```python
from build123d import *

# Parameters (mm, degrees)
SKETCH1_R           = 5
SKETCH1_R_2         = 3
SKETCH1_W           = 45.892135624
SKETCH1_H           = 6.35
BOSS_EXTRUDE1_DEPTH = 6.35
SKETCH2_R           = 1.5
CUT_EXTRUDE1_DEPTH  = 28.889427262


with BuildPart() as part:
    # Sketch1 → Boss-Extrude1 (new body)
    # profile 1 of 5: a face of its own
    with BuildSketch(Plane.XY):
        Circle(SKETCH1_R)
        Circle(SKETCH1_R_2, mode=Mode.SUBTRACT)
    # profile 2 of 5: a face of its own
    with BuildSketch(Plane.XY):
        with BuildLine():
            ThreePointArc((-4.582078525, -2.001138774), (-4.913002543, 0.92865818), (-3.535533906, 3.535533906))
            Line((-3.535533906, 3.535533906), (-16.596067812, -9.525))
            Line((-16.596067812, -9.525), (-12.105939751, -9.525))
            Line((-12.105939751, -9.525), (-4.582078525, -2.001138774))
        make_face()
    # profile 3 of 5: a face of its own
    with BuildSketch(Plane.XY):
        with Locations((0, -12.7)):
            Rectangle(SKETCH1_W, SKETCH1_H)
    # profile 4 of 5: a face of its own
    with BuildSketch(Plane.XY):
        with BuildLine():
            ThreePointArc((1.5875, -4.741291359), (0, -5), (-1.5875, -4.741291359))
            Line((-1.5875, -4.741291359), (-1.5875, -9.525))
            Line((-1.5875, -9.525), (1.5875, -9.525))
            Line((1.5875, -9.525), (1.5875, -4.741291359))
        make_face()
    # profile 5 of 5: a face of its own
    with BuildSketch(Plane.XY):
        with BuildLine():
            Line((16.596067812, -9.525), (3.535533906, 3.535533906))
            ThreePointArc((3.535533906, 3.535533906), (4.619397663, 1.913417162), (5, 0))
            ThreePointArc((5, 0), (4.894404592, -1.022156391), (4.582078525, -2.001138774))
            Line((4.582078525, -2.001138774), (12.105939751, -9.525))
            Line((12.105939751, -9.525), (16.596067812, -9.525))
        make_face()
    extrude(amount=BOSS_EXTRUDE1_DEPTH)

    # Sketch2 → Cut-Extrude1 (cut, through all)
    with BuildSketch(Plane(origin=(0, -9.525, 0), x_dir=(1, 0, 0), z_dir=(0, 1, 0))):
        with Locations(Location((19.771067812, -3.175, 0), (0, 0, 270))):
            Circle(SKETCH2_R)
        with Locations(Location((-19.771067812, -3.175, 0), (0, 0, 270))):
            Circle(SKETCH2_R)
    extrude(amount=-CUT_EXTRUDE1_DEPTH, mode=Mode.SUBTRACT)


solid = part.part
```
Input: part model. Units: mm. Frame: model coordinates. A direction names the side the tool comes from. Coordinates: 2 decimals unless noted, no trailing zeros. Write each loop counter-clockwise with the first axis right and the second up, starting at its lowest first coordinate (ties: lowest second). Pieces come first, ordered by that corner, then holes. Notation, with made-up numbers: M 54,-23.5 L 74,-23.5 A25 cw 74,-4.5 Z; hole C -13,39.5 d10. An arc over 180 degrees is marked long. Use one line per item in the form item = value.
Q1. Section C-C (y = 0). Return loops of the section in (x, z).
Answer below:
outline = M -7.07,0 L -3,0 L -3,6.35 L -7.07,6.35 Z; M 3,0 L 7.07,0 L 7.07,6.35 L 3,6.35 Z
Q2. Section D-D (y = -12.25). Return loops of the section in (x, z) (3 decimals), plus the area to 3 significant figures.
Answer below:
outline = M -22.946,0 L 22.946,0 L 22.946,6.35 L -22.946,6.35 Z; hole C -19.771,3.175 d3; hole C 19.771,3.175 d3
area = 277 mm²
Q3. Set-up query: faces 1 (the face through (8.29, -5.71, 3.13)), 2 (the face through (22.946, -13, 3)), 3 (the face through (19, -9.525, 5)). Return all of +Z, -Z, +X, -X, +Y, -Y with unobstructed straight access to the full face (end or side cutting, diameter ignored); none if empty.
Answer below:
face_1 = +Z, -Z
face_2 = +Z, -Z, +X, +Y, -Y
face_3 = +Z, -Z, +X, +Y
Q4. First-contact query: pin 1 (1.4 mm diameter, centred on y = -6.5, z = 4.5, fed in from -X); pin 2 (1.9 mm diameter, centred on x = -19, z = 3.5, fed in from +Y) (3 decimals); pin 3 (8 mm diameter, centred on x = 1, y = 0, fed in from +Z); pin 4 (1.9 mm diameter, centred on x = 7, z = 4, fed in from +Y). Flat tips, straight axial feed; report the tip coordinate or a pass-through.
Answer below:
pin_1 = -14.27
pin_2 = -9.525
pin_3 = 6.35
pin_4 = 1.02
Q5. Section A-A (x = -5.5). Return loops of the section in (y, z) (3 decimals).
Answer below:
outline = M -15.875,0 L -9.525,0 L -9.525,6.35 L -15.875,6.35 Z; M -2.919,0 L 1.571,0 L 1.571,6.35 L -2.919,6.35 Z
Q6. Section B-B (z = 3.5). Return loops of the section in (x, y) (1 decimal), plus the area to 3 significant figures.
Answer below:
outline = M -22.9,-15.9 L -21.2,-15.9 L -21.2,-9.5 L -22.9,-9.5 Z; M -18.3,-15.9 L 18.3,-15.9 L 18.3,-9.5 L 16.6,-9.5 L 3.5,3.5 A5 ccw -3.5,3.5 L -16.6,-9.5 L -18.3,-9.5 Z; M 21.2,-15.9 L 22.9,-15.9 L 22.9,-9.5 L 21.2,-9.5 Z; hole M -12.1,-9.5 L -1.6,-9.5 L -1.6,-4.7 A5 cw -4.6,-2 Z; hole C 0,0 d6; hole M 1.6,-9.5 L 12.1,-9.5 L 4.6,-2 A5 cw 1.6,-4.7 Z
area = 405 mm²
Q7. Material intervals for probe 1 along X at (y, z) = (-14.25, 3.75); probe 2 along X at (y, z) = (-12.75, 4.5); probe 3 along Y at (x, z) = (0, 2.5) (3 decimals), sorted ascending. Write a range as from..to.
Answer below:
probe_1 = -22.95..-21.16, -18.39..18.39, 21.16..22.95
probe_2 = -22.95..-20.47, -19.07..19.07, 20.47..22.95
probe_3 = -15.875..-3, 3..5
Q8. Draft query along X for faces 4 (the face through (-18, -9.525, 4)), 5 (the face through (-22.946, -13, 3)), 6 (the face through (-8.4, -5.82, 3.13)). Return one class per face: released by +X, released by -X, zero draft, split by the parting line, or undercut.
Answer below:
face_4 = zero draft
face_5 = released by -X
face_6 = undercut
